Work out the finished part from the listing and answer in its coordinate system (mm). A direction names the side the tool comes from. Coordinates: 2 decimals unless noted, no trailing zeros. Order: outer loops, then holes, each group sorted by start corner. A loop starts at its lowest first (then second) coordinate and runs counter-clockwise, first axis right, second up. Notation, with made-up numbers: (59.5, 27.25) -> (86.5, 27.25) arc R35 cw to (86.5, 59.25) -> close; hole circle Ø9 at (29.5, 13.25). An arc over 180 degrees is marked (long way). Use one line per item in the form item = value.
from build123d import *

# Parameters (mm, degrees)
SKETCH1_R             = 2.6162
BOSS_EXTRUDE1_DEPTH   = 2.54
BOSS_EXTRUDE1_2_DEPTH = 2.54
BOSS_EXTRUDE2_DEPTH   = 12.7
BOSS_EXTRUDE3_DEPTH   = 12.7
CUT_EXTRUDE1_DEPTH    = 10.16
BOSS_EXTRUDE5_DEPTH   = 12.7
CUT_EXTRUDE2_DEPTH    = 10.16


with BuildPart() as part:
    # Sketch1 → Boss-Extrude1 (new body)
    with BuildSketch(Plane(origin=(0, 0, 0), x_dir=(1, 0, 0), z_dir=(0, 1, 0))):
        with BuildLine():
            Line((-10.149829081, -0.78559745), (-12.970179614, -5.786096043))
            ThreePointArc((-12.970179614, -5.786096043), (-14.833663899, -11.850889023), (-9.017306722, -14.385504725))
            Line((-9.017306722, -14.385504725), (-1.886569513, -12.038188494))
            Line((-1.886569513, -12.038188494), (-10.149829081, -0.78559745))
        make_face()
        with Locations((-10.506432822, -9.861799418)):
            Circle(SKETCH1_R, mode=Mode.SUBTRACT)
    extrude(amount=BOSS_EXTRUDE1_DEPTH)



with BuildPart() as body_2:
    # Sketch1 → Boss-Extrude1 2 (new body)
    with BuildSketch(Plane(origin=(0, 0, 0), x_dir=(1, 0, 0), z_dir=(0, 1, 0))):
        with BuildLine():
            Line((5.95620443, 11.428082994), (14.562195858, 0.435395631))
            Line((14.562195858, 0.435395631), (18.746273034, 6.66843701))
            ThreePointArc((18.746273034, 6.66843701), (18.171308738, 12.678699935), (12.165175551, 13.29531044))
            Line((12.165175551, 13.29531044), (5.95620443, 11.428082994))
        make_face()
        with Locations((14.792061634, 9.322795398)):
            Circle(SKETCH1_R, mode=Mode.SUBTRACT)
    extrude(amount=BOSS_EXTRUDE1_2_DEPTH)


with BuildPart() as part_1:
    add(part.part)

    add(body_2.part)  # Boss-Extrude2 merges body 2
    # Sketch1<5> → Boss-Extrude2 (add)
    with BuildSketch(Plane(origin=(0, 0, 0), x_dir=(1, 0, 0), z_dir=(0, 1, 0))):
        with BuildLine():
            Line((-10.256120569, 2.902434291), (-10.149829081, -0.78559745))
            Line((-10.149829081, -0.78559745), (-1.886569513, -12.038188494))
            Line((-1.886569513, -12.038188494), (-0.005832357, -11.419082121))
            Line((-0.005832357, -11.419082121), (-4.572272753, -5.200678127))
            ThreePointArc((-4.572272753, -5.200678127), (-5.731382948, -2.990882077), (-6.18409173, -0.536948544))
            Line((-6.18409173, -0.536948544), (-6.647421935, 0.770957563))
            Line((-6.647421935, 0.770957563), (-12.168687381, 8.289605816))
            Line((-12.168687381, 8.289605816), (-1.892547948, 15.835815142))
            Line((-1.892547948, 15.835815142), (3.512453439, 8.475490841))
            Line((3.512453439, 8.475490841), (4.646859497, 7.676481354))
            ThreePointArc((4.646859497, 7.676481354), (6.992594353, 6.504605156), (8.857901564, 4.661674107))
            Line((8.857901564, 4.661674107), (13.456324189, -1.212027104))
            Line((13.456324189, -1.212027104), (14.562195858, 0.435395631))
            Line((14.562195858, 0.435395631), (5.95620443, 11.428082994))
            Line((5.95620443, 11.428082994), (2.433604251, 12.525427051))
            Line((2.433604251, 12.525427051), (-0.436996693, 16.310853991))
            Line((-0.436996693, 16.310853991), (-3.639779121, 16.751054765))
            Line((-3.639779121, 16.751054765), (-12.686520738, 9.890643659))
            Line((-12.686520738, 9.890643659), (-13.126721512, 6.687861232))
            Line((-13.126721512, 6.687861232), (-10.256120569, 2.902434291))
        make_face()
    extrude(amount=BOSS_EXTRUDE2_DEPTH)

    # Sketch1<6> → Boss-Extrude3 (add)
    with BuildSketch(Plane(origin=(0, 0, 0), x_dir=(1, 0, 0), z_dir=(0, 1, 0))):
        with BuildLine():
            Line((-6.647421935, 0.770957563), (-6.18409173, -0.536948544))
            ThreePointArc((-6.18409173, -0.536948544), (7.176852085, -6.907826955), (4.646859497, 7.676481354))
            Line((4.646859497, 7.676481354), (3.512453439, 8.475490841))
            Line((3.512453439, 8.475490841), (-1.892547948, 15.835815142))
            Line((-1.892547948, 15.835815142), (-12.168687381, 8.289605816))
            Line((-12.168687381, 8.289605816), (-6.647421935, 0.770957563))
        make_face()
    extrude(amount=BOSS_EXTRUDE3_DEPTH)

    # Sketch1<8> → Cut-Extrude1 (cut)
    with BuildSketch(Plane(origin=(0, 0, 0), x_dir=(1, 0, 0), z_dir=(0, 1, 0))):
        with BuildLine():
            Line((-6.647421935, 0.770957563), (-6.18409173, -0.536948544))
            ThreePointArc((-6.18409173, -0.536948544), (7.176852085, -6.907826955), (4.646859497, 7.676481354))
            Line((4.646859497, 7.676481354), (3.512453439, 8.475490841))
            Line((3.512453439, 8.475490841), (-1.892547948, 15.835815142))
            Line((-1.892547948, 15.835815142), (-12.168687381, 8.289605816))
            Line((-12.168687381, 8.289605816), (-6.647421935, 0.770957563))
        make_face()
    extrude(amount=CUT_EXTRUDE1_DEPTH, mode=Mode.SUBTRACT)

    # Sketch1<9> → Boss-Extrude5 (add)
    with BuildSketch(Plane(origin=(0, 0, 0), x_dir=(1, 0, 0), z_dir=(0, 1, 0))):
        with BuildLine():
            Line((-4.572272753, -5.200678127), (-0.005832357, -11.419082121))
            Line((-0.005832357, -11.419082121), (5.244167697, -9.690872263))
            Line((5.244167697, -9.690872263), (10.378118681, -5.797645747))
            Line((10.378118681, -5.797645747), (13.456324189, -1.212027104))
            Line((13.456324189, -1.212027104), (8.857901564, 4.661674107))
            ThreePointArc((8.857901564, 4.661674107), (7.073990523, -6.984589168), (-4.572272753, -5.200678127))
        make_face()
    extrude(amount=BOSS_EXTRUDE5_DEPTH)

    # Sketch1<11> → Cut-Extrude2 (cut)
    with BuildSketch(Plane(origin=(0, 0, 0), x_dir=(1, 0, 0), z_dir=(0, 1, 0))):
        with BuildLine():
            Line((-4.572272753, -5.200678127), (-0.005832357, -11.419082121))
            Line((-0.005832357, -11.419082121), (5.244167697, -9.690872263))
            Line((5.244167697, -9.690872263), (10.378118681, -5.797645747))
            Line((10.378118681, -5.797645747), (13.456324189, -1.212027104))
            Line((13.456324189, -1.212027104), (8.857901564, 4.661674107))
            ThreePointArc((8.857901564, 4.661674107), (7.073990523, -6.984589168), (-4.572272753, -5.200678127))
        make_face()
    extrude(amount=CUT_EXTRUDE2_DEPTH, mode=Mode.SUBTRACT)


solid = part_1.part
(1) Section B-B on z = 10.5 is taken. Write down the section's boundary in (x, y), plus the area to 3 significant figures.
Data:
outline = (-15.23, 0) -> (-13.04, 0) -> (-13.04, 2.54) -> (-15.23, 2.54) -> close; (-7.97, 0) -> (-0.68, 0) -> (-0.68, 10.16) -> (2.79, 10.16) -> (2.79, 12.7) -> (-3.02, 12.7) -> (-3.02, 2.54) -> (-7.97, 2.54) -> close
area = 56.6 mm²
(2) Straight lines are drawn through the part: line 1 along Y through (x, z) = (-1, 3.5); line 2 along Y through (x, z) = (15.5, -4); line 3 along X through (y, z) = (1.25, 0). For each, find the intervals that lie inside material, in ascending order.
Data:
line_1 = 10.16 to 12.7
line_2 = 0 to 2.54
line_3 = -10.17 to -6.37, 12.51 to 14.27
(3) Section A-A on y = 10.75 is taken. Write down the section's boundary in (x, z).
Data:
outline = (-13.13, -6.69) -> (-12.69, -9.89) -> (-3.64, -16.75) -> (-0.44, -16.31) -> (2.43, -12.53) -> (5.96, -11.43) -> (14.56, -0.44) -> (10.38, 5.8) -> (5.24, 9.69) -> (-1.89, 12.04) -> (-10.15, 0.79) -> (-10.26, -2.9) -> close
(4) Each of these flat-tipped pins is pushed along its axis until it touches: P1, Ø1, axis at x = -3.5, y = 2, coming from the -Z side; P2, Ø4, axis at x = 13.5, z = -5.5, coming from the +Y side; P3, Ø1.5, axis at y = 3.5, z = -7.5, coming from the +X side; P4, Ø1, axis at x = 0, y = 7.5, coming from the +Z side. Where does it stop, or does it pass through?
Data:
P1 = -16.75
P2 = 2.54
P3 = 9.62
P4 = 11.58
(5) Section D-D on y = 2 is taken. Write down the section's boundary in (x, z) (1 decimal), plus the area to 3 significant figures.
Data:
outline = (-13.1, -6.7) -> (-12.7, -9.9) -> (-3.6, -16.8) -> (-0.4, -16.3) -> (2.4, -12.5) -> (6, -11.4) -> (12.2, -13.3) arc R4.8 ccw to (18.7, -6.7) -> (13.5, 1.2) -> (8.9, -4.7) arc R8.3 cw to (4.6, -7.7) -> (3.5, -8.5) -> (-1.9, -15.8) -> (-12.2, -8.3) -> (-6.6, -0.8) -> (-6.2, 0.5) arc R8.3 cw to (-4.6, 5.2) -> (0, 11.4) -> (-9, 14.4) arc R4.8 ccw to (-13, 5.8) -> (-10.1, 0.8) -> (-10.3, -2.9) -> close; hole circle Ø5.2 at (-10.5, 9.9); hole circle Ø5.2 at (14.8, -9.3)
area = 283 mm²
(6) Which of the six approach directions +Z, -Z, +X, -X, +Y, -Y give full straight-line access (tool end or side, diameter ignored) to faces 1 (the flat face through (-6.1, 7.5, 6.3)), 2 (the flat face through (-2.32, 5.01, 8.27)), 3 (the flat face through (-6.42, 5.01, -0.13))?
Data:
face_1 = +Z, -X, +Y
face_2 = +X, -Y
face_3 = -Y
(7) Section C-C on x = 15 is taken. Write down the section's boundary in (y, z), plus the area to 3 significant figures.
Data:
outline = (0, -14.08) -> (2.54, -14.08) -> (2.54, -11.93) -> (0, -11.93) -> close; (0, -6.71) -> (2.54, -6.71) -> (2.54, -1.09) -> (0, -1.09) -> close
area = 19.8 mm²
(8) The mould has two halves that part along Z. Classify faces 4 (the flat face through (4.09, 5.01, -8.07)), 5 (the flat face through (-6.959, 5.009, -12.116)), 6 (the flat face through (1.02, 6.26, -14.39)), 7 (the flat face through (0.85, 5.01, -12.1)): released by +Z, released by -Z, zero draft, split by the parting line, or undercut.
Data:
face_4 = released by +Z
face_5 = undercut
face_6 = released by -Z
face_7 = undercut
